Source: three-view drawing plus pictorial views. Frame: mm from the lowest corner of the part. A direction names the side the tool comes from. Give positions to 0.01 mm unless a question says otherwise; leave off trailing zeros. Order: outer loops, then holes, each group sorted by start corner. A loop starts at its lowest first (then second) coordinate and runs counter-clockwise, first axis right, second up.
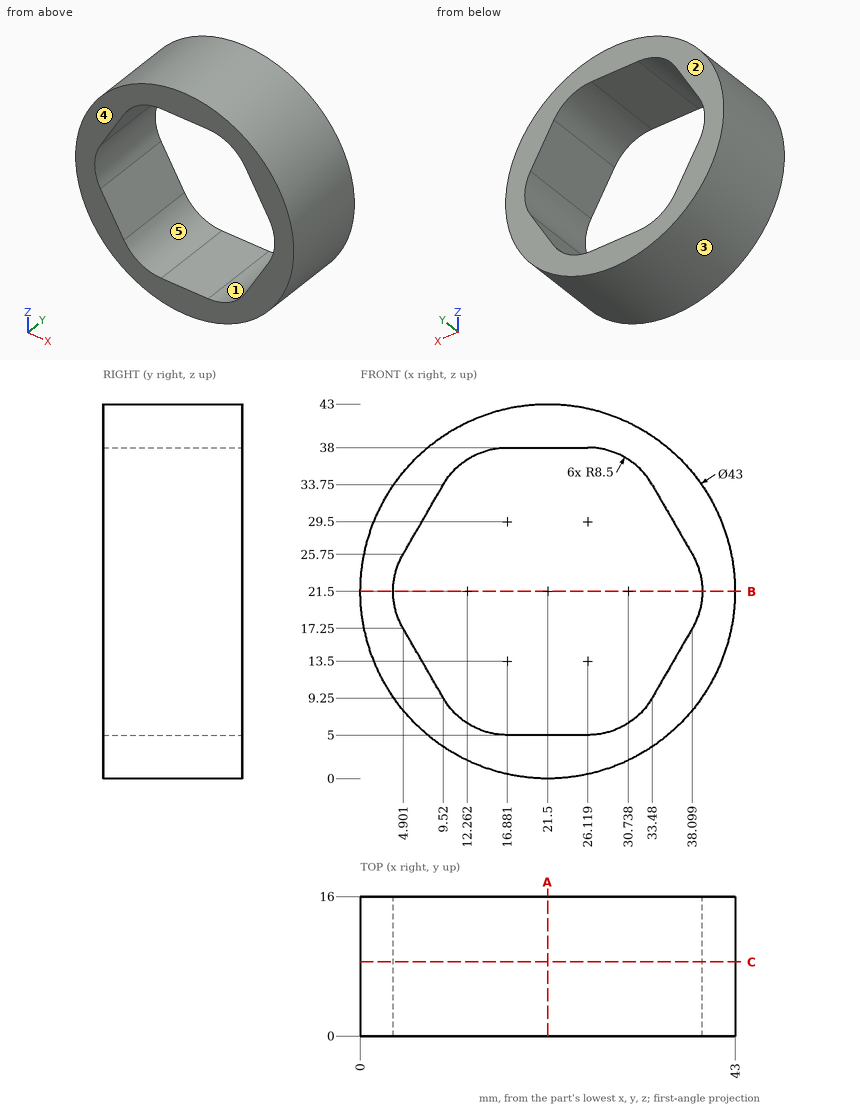
(1) Section B-B, the plane z = 21.5. Return loops of the section in (x, y).
(2) Draft query along Z for the marked faces 1, 2 and 3. Return one class per face: +Z half, -Z half, draft (parallel to the pull), parting line (faces both ways), or undercut.
(3) Access query for the marked faces 4 and 5. Directions: +Z, -Z, +X, -X, +Y, -Y. A direction counts if a zero-diameter tool reaches every point of the face in a straight line with its end or side. Return the directions, or none.
(4) Section A-A, the plane x = 21.5. Return loops of the section in (y, z), plus the area to 3 significant figures.
(5) Pin query (flat end, axial travel): pin 1 Ø1 at (y, z) = (3, 9) entering from +X; pin 2 Ø4 at (y, z) = (12, 11.5) entering from -X; pin 3 Ø1.5 at (y, z) = (9, 29) entering from -X. Return the tip coordinate at first contact, or that it passes through.
(6) Line query: line 1 along Z through (x, y) = (21, 1.25) (1 decimal); line 2 along X through (y, z) = (9.5, 34); line 3 along X through (y, z) = (13.5, 24) (1 decimal). Output: solid intervals per line, ascending.
(7) Section C-C, the plane y = 8.5. Return loops of the section in (x, z).
Checks:
1. outline: (0, 0) - (3.76, 0) - (3.76, 16) - (0, 16) - close; (39.24, 0) - (43, 0) - (43, 16) - (39.24, 16) - close
2. face 1: undercut
2. face 2: draft
2. face 3: parting line
3. face 4: +Z, -Z, +X, -X, -Y
3. face 5: +Y, -Y
4. outline: (0, 0) - (16, 0) - (16, 5) - (0, 5) - close; (0, 38) - (16, 38) - (16, 43) - (0, 43) - close
4. area: 160 mm2
5. pin 1: stops at x = 39.34
5. pin 2: stops at x = 1.54
5. pin 3: stops at x = 1.09
6. line 1: z = 0 to 5, 38 to 43
6. line 2: x = 4.01 to 9.67, 33.33 to 38.99
6. line 3: x = 0.1 to 4.1, 38.9 to 42.9
7. outline: circle Ø43 at (21.5, 21.5); hole (4.9, 17.25) - (9.52, 9.25) arc R8.5 ccw to (16.88, 5) - (26.12, 5) arc R8.5 ccw to (33.48, 9.25) - (38.1, 17.25) arc R8.5 ccw to (38.1, 25.75) - (33.48, 33.75) arc R8.5 ccw to (26.12, 38) - (16.88, 38) arc R8.5 ccw to (9.52, 33.75) - (4.9, 25.75) arc R8.5 ccw to start
